Source: CAD feature listing. Evaluate the final solid. Frame: model axes, mm. A direction names the side the tool comes from. Give positions to 0.01 mm unless a question says otherwise; leave off trailing zeros. Loops run counter-clockwise (first coordinate to the right, second up) from the corner with the lowest first, then second, coordinate; pieces in that order, holes last. Notation, with made-up numbers: (64, 35.25) - (90, 35.25) arc R16 ccw to (90, 50.25) - close; hole circle Ø4 at (-38, -7). An arc over 180 degrees is marked (long way). Put each result on its own line as item: value.
```python
from build123d import *

# Parameters (mm, degrees)
F0_R     = 3.175
F1_DEPTH = 6.35
F5_DEPTH = 25.4
F7_DEPTH = 5.08
F8_DEPTH = 25.4


# Not quite as in the source:
# - the program builds the solid bodies; features that only make, move or delete a surface that nothing else refers to are left out


with BuildPart() as f1:
    # F0 (on Right) → F1 (new body)
    with BuildSketch(Plane.YZ):
        with Locations((-37.7712212503, 38.5835021734)):
            Circle(F0_R)
    extrude(amount=F1_DEPTH)

    # F4 (on face) → F5 (join)
    with BuildSketch(Plane.YZ.offset(6.35)):
        with BuildLine():
            ThreePointArc((-34.5962212503, 38.5835021734), (-35.5085896731, 40.8108601029), (-37.7213383186, 41.7581102899))
            Line((-37.7213383186, 41.7581102899), (-37.7712212503, 38.5835021734))
            Line((-37.7712212503, 38.5835021734), (-34.5966131338, 38.5336192417))
            ThreePointArc((-34.5966131338, 38.5336192417), (-34.5963192227, 38.5585599379), (-34.5962212503, 38.5835021734))
        make_face()
    extrude(amount=F5_DEPTH)

    # F6 (on face) → F7 (join)
    with BuildSketch(Plane.YZ.offset(31.75)):
        Polygon((-37.7712212503, 38.5835021734), (-36.1839171921, 38.5585607076), (-36.1610525797, 40.0136913835), (-36.1610525797, 40.1458973996), (-37.7462797844, 40.1708062317), align=None)
    extrude(amount=F7_DEPTH)

    # F8 (add): a face of the model
    f8_faces = [f1.faces().sort_by_distance(p)[0] for p in [
        (34.29, -36.953666182, 40.1583518156),
    ]]
    extrude(f8_faces, amount=F8_DEPTH)


solid = f1.part
```
1) Section query B-B, the plane y = -40.25. Output: boundary loops of the cut face in (x, z), plus the area to 3 significant figures.
Check result:
outline: (0, 36.6) - (6.35, 36.6) - (6.35, 40.57) - (0, 40.57) - close
area: 25.2 mm²
2) Section query A-A, the plane x = 34.5. Output: boundary loops of the cut face in (y, z), plus the area to 3 significant figures.
Check result:
outline: (-37.77, 38.58) - (-36.18, 38.56) - (-36.16, 40.01) - (-36.16, 40.15) - (-35.76, 65.54) - (-37.35, 65.57) - close
area: 42.8 mm²
3) Access query for faces 1 (the flat face through (36.83, -37, 52)), 2 (the flat face through (31.75, -36, 40)). Directions: +Z, -Z, +X, -X, +Y, -Y. A direction counts if a zero-diameter tool reaches every point of the face in a straight line with its end or side. Return the directions, or none.
Check result:
face 1: +Z, -Z, +X, +Y, -Y
face 2: -Z, +X, +Y
4) Material intervals for line 1 along X through (y, z) = (-37, 46); line 2 along X through (y, z) = (-35.75, 39); line 3 along Z through (x, y) = (28.5, -36), sorted ascending. Write a range as [from, to].
Check result:
line 1: [31.75, 36.83]
line 2: [0, 31.75]
line 3: [38.56, 41.22]
5) Pin query (flat end, axial travel): P1, Ø1.6, axis at y = -36.5, z = 58.5, coming from the -X side. Return the tip coordinate at first contact, or that it passes through.
Check result:
P1: x = 31.75
